Model file for the job. Use its own axes, mm. A direction names the side the tool comes from. Coordinates: 2 decimals unless noted, no trailing zeros. Order: outer loops, then holes, each group sorted by start corner. A loop starts at its lowest first (then second) coordinate and runs counter-clockwise, first axis right, second up. Notation, with made-up numbers: (55.5, 84.5) -> (79.5, 84.5) arc R17 ccw to (79.5, 95.5) -> close; hole circle Ø10 at (68.25, 34). An arc over 180 degrees is marked (long way). Use CSV: the item, a comma, the result in double quotes. Start each with the question number.
(1) Probe L1, parallel to X at y = 0, z = 1.5; L2, parallel to Z at x = 113.5, y = 4.5; L3, parallel to X at y = 0.75, z = 0.3. List the from-to ranges inside material, lowest first.
(2) Pin check, flat tips, straight feed: pin 1 Ø5 at (x, y) = (117.5, 1) entering from -Z; pin 2 Ø2 at (x, z) = (90.5, 4.5) entering from +Y; pin 3 Ø0.9 at (y, z) = (3.5, 2) entering from +X; pin 4 Ø1 at (y, z) = (-3.5, 3.5) entering from -X. Stop position of each tip, or through.
(3) Cut at A-A on z = 1.5. Write the cut outline in (x, y), plus the area to 3 significant figures.
(4) Tool access for faces 1 (the cylindrical face through (71.96, 6.6, 5.14)), 2 (the flat face through (1.5, 0, 1)): list every direction of +Z, -Z, +X, -X, +Y, -Y with a clear straight run to the whole face (end or side of a thin tool).
```python
from build123d import *

# Parameters (mm, degrees)
SKETCH_1_W          = 3
SKETCH_1_H          = 15
EXTRUDE_1_DEPTH     = 6
SKETCH_2_W          = 3
SKETCH_2_H          = 15
EXTRUDE_2_DEPTH     = 146
SKETCH_3_R          = 1
CUT_EXTRUDE_1_DEPTH = 146
FILLET_1_R          = 3


with BuildPart() as part:
    # 草图1 → 凸台-拉伸1 (new body)
    with BuildSketch(Plane.XY):
        Rectangle(SKETCH_1_W, SKETCH_1_H)
    extrude(amount=EXTRUDE_1_DEPTH)

    # 草图2 → 凸台-拉伸2 (add)
    with BuildSketch(Plane(origin=(1.5, 0, 0), x_dir=(0, 0, -1), z_dir=(1, 0, 0))):
        with Locations((-4.5, 0)):
            Rectangle(SKETCH_2_W, SKETCH_2_H)
    extrude(amount=EXTRUDE_2_DEPTH)

    # 草图3 → 切除-拉伸1 (cut)
    with BuildSketch(Plane(origin=(0, 7.5, 0), x_dir=(1, 0, 0), z_dir=(0, 1, 0))):
        with Locations(Location((0, -1.5, 0), (0, 0, 270))):
            Circle(SKETCH_3_R)
    extrude(amount=-CUT_EXTRUDE_1_DEPTH, mode=Mode.SUBTRACT)

    # 圆角1
    fillet_1_edges = [part.edges().sort_by_distance(p)[0] for p in [
        (-1.5, 0, 6),
        (73, 7.5, 6),
        (147.5, 0, 6),
        (73, -7.5, 6),
    ]]
    fillet(fillet_1_edges, radius=FILLET_1_R - 0.0001)  # a hair under: the kernel refuses the full size


solid = part.part
```
Outcome:
1,L1,"-1.5 to -1, 1 to 1.5"
1,L2,"3 to 6"
1,L3,"-1.5 to 1.5"
2,pin 1,"z = 3"
2,pin 2,"y = 7.46"
2,pin 3,"x = 1.5"
2,pin 4,"x = -1.5"
3,outline,"(-1.5, -7.5) -> (-1, -7.5) -> (-1, 7.5) -> (-1.5, 7.5) -> close; (1, -7.5) -> (1.5, -7.5) -> (1.5, 7.5) -> (1, 7.5) -> close"
3,area,"15.0 mm2"
4,face 1,"+Z, +X, -X, +Y"
4,face 2,"-Z, +X, +Y, -Y"
